The model under review builds one solid part; all positions refer to its coordinate system, in mm. Coordinates: 2 decimals unless noted, no trailing zeros. Order: outer loops, then holes, each group sorted by start corner. A loop starts at its lowest first (then second) coordinate and runs counter-clockwise, first axis right, second up. Notation, with made-up numbers: M 87,-20 L 146,-20 A22 cw 146,15 Z; hole C 4.5,86 d3. An arc over 180 degrees is marked long. Answer in a Markdown table with one row per item.
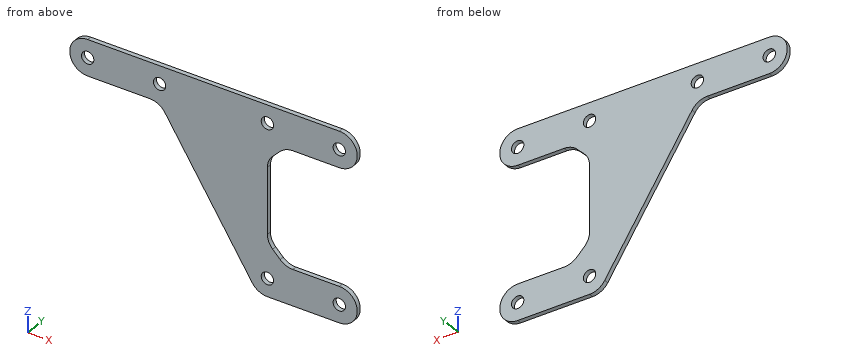
Autodesk Inventor part; units mm, degrees
ref_plane "YZ Plane" through (0, 0, 0) normal (1, 0, 0) x (0, 1, 0)
ref_plane "XZ Plane" through (0, 0, 0) normal (0, 1, 0) x (-1, 0, 0)
ref_plane "XY Plane" through (0, 0, 0) normal (0, 0, 1) x (1, 0, 0)
sketch "main" plane through (0, 0, 0) normal (0, 0, 1) x (1, 0, 0)
  circle A0 centre (-18.4512, -23.1863) radius 2.1844
  line L0 (-22.9413, -14.9764) -> (-20.311, -12.3462)
  line L1 (-43.8512, -16.8363) -> (-27.4314, -16.8363)
  arc A1 (-27.4314, -16.8363) -> (-22.9413, -14.9764) centre (-27.4314, -10.4863) ccw
  circle A2 centre (-43.8512, -23.1863) radius 2.1844
  arc A3 (-43.8512, -16.8363) -> (-43.8512, -29.5363) centre (-43.8512, -23.1863) ccw
  arc A4 (-20.311, -12.3462) -> (-18.4512, -7.856) centre (-24.8012, -7.856) ccw
  line L2 (-18.4512, 15.4585) -> (-18.4512, -7.856)
  line L3 (17.7748, 21.5177) -> (-13.1066, -26.6153)
  arc A5 (-18.4512, 15.4585) -> (-20.311, 19.9486) centre (-24.8012, 15.4585) ccw
  line L4 (-22.9413, 22.5788) -> (-20.311, 19.9486)
  arc A6 (-22.9413, 22.5788) -> (-27.4314, 24.4387) centre (-27.4314, 18.0887) ccw
  circle A7 centre (-43.8512, 30.7887) radius 2.1844
  circle A8 centre (-18.4512, 30.7887) radius 2.1844
  circle A9 centre (19.6488, 30.7887) radius 2.1844
  line L5 (45.0488, 37.1387) -> (-43.8512, 37.1387)
  line L6 (-27.4314, 24.4387) -> (-43.8512, 24.4387)
  arc A10 (-43.8512, 37.1387) -> (-43.8512, 24.4387) centre (-43.8512, 30.7887) ccw
  arc A11 (23.1193, 24.4387) -> (17.7748, 21.5177) centre (23.1193, 18.0887) ccw
  line L7 (45.0488, 24.4387) -> (23.1193, 24.4387)
  circle A12 centre (45.0488, 30.7887) radius 2.1844
  arc A13 (45.0488, 24.4387) -> (45.0488, 37.1387) centre (45.0488, 30.7887) ccw
  line L8 (-18.4512, -29.5363) -> (-43.8512, -29.5363)
  arc A14 (-18.4512, -29.5363) -> (-13.1066, -26.6153) centre (-18.4512, -23.1863) ccw
  point P0 (-14.0637, 6.8091)
  dimension "d0" = 6.35
  dimension "d1" = 6.35
sketch "Sketch1" plane through (0, 0, 0) normal (0, 1, 0) x (-1, 0, 0)
  circle A0 centre (0, -53.975) radius 2.1844
  line L0 (-4.4901, -45.7651) -> (-1.8599, -43.1349)
  line L1 (-25.4, -47.625) -> (-8.9803, -47.625)
  arc A1 (-8.9803, -47.625) -> (-4.4901, -45.7651) centre (-8.9803, -41.275) ccw
  circle A2 centre (-25.4, -53.975) radius 2.1844
  arc A3 (-25.4, -47.625) -> (-25.4, -60.325) centre (-25.4, -53.975) ccw
  arc A4 (-1.8599, -43.1349) -> (0, -38.6447) centre (-6.35, -38.6447) ccw
  line L2 (0, -15.3303) -> (0, -38.6447)
  line L3 (36.2259, -9.271) -> (5.3446, -57.404)
  arc A5 (0, -15.3303) -> (-1.8599, -10.8401) centre (-6.35, -15.3303) ccw
  line L4 (-4.4901, -8.2099) -> (-1.8599, -10.8401)
  arc A6 (-4.4901, -8.2099) -> (-8.9803, -6.35) centre (-8.9803, -12.7) ccw
  circle A7 centre (-25.4, 0) radius 2.1844
  circle A8 centre (0, 0) radius 2.1844
  circle A9 centre (38.1, 0) radius 2.1844
  line L5 (63.5, 6.35) -> (-25.4, 6.35)
  line L6 (-8.9803, -6.35) -> (-25.4, -6.35)
  arc A10 (-25.4, 6.35) -> (-25.4, -6.35) centre (-25.4, 0) ccw
  arc A11 (41.5705, -6.35) -> (36.2259, -9.271) centre (41.5705, -12.7) ccw
  line L7 (63.5, -6.35) -> (41.5705, -6.35)
  circle A12 centre (63.5, 0) radius 2.1844
  arc A13 (63.5, -6.35) -> (63.5, 6.35) centre (63.5, 0) ccw
  line L8 (0, -60.325) -> (-25.4, -60.325)
  arc A14 (0, -60.325) -> (5.3446, -57.404) centre (0, -53.975) ccw
extrude "Extrusion1" add sketch "Sketch1" along normal blind 1.5875
properties part number "gusset" material "Acetal Resin, White"
(1) Take a section at B-B (x = -38.1). Write out the cut boundary in (y, z), then the cut area to 3 significant figures.
Report:
| item | result |
|---|---|
| outline | M 0,-7.38 L 1.59,-7.38 L 1.59,-2.18 L 0,-2.18 Z; M 0,2.18 L 1.59,2.18 L 1.59,6.35 L 0,6.35 Z |
| area | 14.9 mm^2 |
(2) Take a section at C-C (y = 0.3). State how many separate pieces and enclosed holes the cut face has, then the cut area to 3 significant figures.
Report:
| item | result |
|---|---|
| separate pieces | 1 |
| enclosed holes | 6 |
| area | 2,720 mm^2 |
(3) To check wall thickness, follow line 1 (Z direction, x = 25.5, y = 0.75); line 2 (X direction, y = 0.6, z = 1.5); line 3 (Z direction, x = 28.5, y = 0.25). State the ranges of each line that lie inside material, in increasing order. Write a range as [from, to].
Report:
| item | result |
|---|---|
| line 1 | [-60.32, -56.16], [-51.79, -47.63], [-6.35, -2.18], [2.18, 6.35] |
| line 2 | [-69.67, -65.09], [-61.91, -39.69], [-36.51, -1.59], [1.59, 23.81], [26.99, 31.57] |
| line 3 | [-59.52, -48.43], [-5.54, 5.54] |
(4) Take a section at D-D (z = -41.5). Write out the cut boundary in (x, y).
Report:
| item | result |
|---|---|
| outline | M -15.55,0 L 0.68,0 L 0.68,1.59 L -15.55,1.59 Z |
(5) Take a section at A-A (z = 0). Write out the cut boundary in (x, y).
Report:
| item | result |
|---|---|
| outline | M -69.85,0 L -65.68,0 L -65.68,1.59 L -69.85,1.59 Z; M -61.32,0 L -40.28,0 L -40.28,1.59 L -61.32,1.59 Z; M -35.92,0 L -2.18,0 L -2.18,1.59 L -35.92,1.59 Z; M 2.18,0 L 23.22,0 L 23.22,1.59 L 2.18,1.59 Z; M 27.58,0 L 31.75,0 L 31.75,1.59 L 27.58,1.59 Z |
